CAD build for the part. Positions are in the model's coordinates, mm. A direction names the side the tool comes from. Round coordinates to 2 decimals unless told otherwise and drop trailing zeros. Loops run counter-clockwise (first coordinate to the right, second up) from the corner with the lowest first, then second, coordinate; pieces in that order, holes last.
from build123d import *

# Parameters (mm, degrees)
F0_R         = 1.5
F0_W         = 21
F0_H         = 8
F0_W_2       = 3
F0_H_2       = 5
F1_DEPTH     = 4
F2_W         = 2
F2_H         = 11
F3_DEPTH     = 1.5
F4_DEPTH     = 8
F5_T1_DEPTH  = 4
F5_T3_DEPTH  = 8
F5_T9_DEPTH  = 20.2494197933
F5_T14_DEPTH = 16.5024140205
F5_T22_DEPTH = 20.2494197933
F5_T27_DEPTH = 16.5024140205


# Not quite as in the source:
# - a fillet or chamfer that OpenCascade refuses, or shapes differently, is made with other operations: its cross-section is extruded or revolved along the edge and cut away or added


with BuildPart() as f1:
    # F0 (on Top) → F1 (new body)
    with BuildSketch(Plane.XY):
        with BuildLine():
            ThreePointArc((-3.25, 9), (0, 5.75), (3.25, 9))
            ThreePointArc((3.25, 9), (0, 12.25), (-3.25, 9))
        make_face()
        with Locations((0, 9)):
            Circle(F0_R, mode=Mode.SUBTRACT)
        with BuildLine():
            Line((3.25, -9), (3.25, 9))
            ThreePointArc((3.25, 9), (0, 5.75), (-3.25, 9))
            Line((-3.25, 9), (-3.25, 4))
            Line((-3.25, 4), (-3.25, -4))
            Line((-3.25, -4), (-3.25, -9))
            ThreePointArc((-3.25, -9), (0, -5.75), (3.25, -9))
        make_face()
        with BuildLine():
            ThreePointArc((-3.25, -9), (0, -12.25), (3.25, -9))
            ThreePointArc((3.25, -9), (0, -5.75), (-3.25, -9))
        make_face()
        with Locations((0, -9)):
            Circle(F0_R, mode=Mode.SUBTRACT)
        with Locations((-13.75, 0)):
            Rectangle(F0_W, F0_H)
        with Locations((-25.75, 0)):
            Rectangle(F0_W_2, F0_H)
        with Locations((-25.75, 6.5)):
            Rectangle(F0_W_2, F0_H_2)
        with Locations((-25.75, -6.5)):
            Rectangle(F0_W_2, F0_H_2)
    extrude(amount=F1_DEPTH)

    # F2 (on face) → F3 (cut)
    with BuildSketch(Plane.XY.offset(4)):
        Rectangle(F2_W, F2_H)
    extrude(amount=-F3_DEPTH, mode=Mode.SUBTRACT)

    # F0 (on Top) → F4 (join)
    with BuildSketch(Plane.XY):
        with Locations((-25.75, 6.5)):
            Rectangle(F0_W_2, F0_H_2)
        with Locations((-25.75, 0)):
            Rectangle(F0_W_2, F0_H)
        with Locations((-25.75, -6.5)):
            Rectangle(F0_W_2, F0_H_2)
    extrude(amount=F4_DEPTH)

    # F5: fillet of radius 5 on 3 edges, made by hand

    # F5_s2 → F5_t1 (join)
    with BuildSketch(Plane.XY):
        with BuildLine():
            ThreePointArc((-19.2490344078, 3.9996), (-22.785192534, 5.4641246619), (-24.2504, 8.9999999228))
            Line((-24.2504, 8.9999999228), (-24.7505365592, 8.9999033465))
            ThreePointArc((-24.7505365592, 8.9999033465), (-24.7501365685, 6.4999999614), (-24.7501365685, 4))
            Line((-24.7501365685, 4), (-24.25, 3.4998634315))
            ThreePointArc((-24.25, 3.4998634315), (-21.7495172039, 3.4998634315), (-19.2490344078, 3.4994634315))
            Line((-19.2490344078, 3.4994634315), (-19.2490344078, 3.9996))
        make_face()
        with BuildLine():
            ThreePointArc((-24.2504, -8.9999999228), (-22.785192534, -5.4641246619), (-19.2490344078, -3.9996))
            Line((-19.2490344078, -3.9996), (-19.2490344078, -3.4994634315))
            ThreePointArc((-19.2490344078, -3.4994634315), (-21.7495172039, -3.4998634315), (-24.25, -3.4998634315))
            Line((-24.25, -3.4998634315), (-24.7501365685, -4))
            ThreePointArc((-24.7501365685, -4), (-24.7501365685, -6.4999999614), (-24.7505365592, -8.9999033465))
            Line((-24.7505365592, -8.9999033465), (-24.2504, -8.9999999228))
        make_face()
    extrude(amount=F5_T1_DEPTH)

    # F5_s4 → F5_t3 (join)
    with BuildSketch(Plane.XZ.offset(-4)):
        with BuildLine():
            ThreePointArc((-19.350232099, 3.9996), (-22.5130680788, 5.126675133), (-24.2503919057, 7.9999199382))
            Line((-24.2503919057, 7.9999199382), (-24.7404078864, 7.8998153635))
            ThreePointArc((-24.7404078864, 7.8998153635), (-24.7501365685, 5.9999599691), (-24.7501365685, 4))
            Line((-24.7501365685, 4), (-24.25, 3.4998634315))
            ThreePointArc((-24.25, 3.4998634315), (-21.8001160495, 3.4998634315), (-19.350232099, 3.4994634315))
            Line((-19.350232099, 3.4994634315), (-19.350232099, 3.9996))
        make_face()
    extrude(amount=F5_T3_DEPTH)


with BuildPart() as f5_tool7:
    # F5_s8 → F5_t9 (new body)
    with BuildSketch(Plane.XZ.offset(-16.2494197933)):
        with BuildLine():
            ThreePointArc((-19.350232099, 3.9996), (-22.5130680788, 5.126675133), (-24.2503919057, 7.9999199382))
            Line((-24.2503919057, 7.9999199382), (-24.7404078864, 7.8998153635))
            ThreePointArc((-24.7404078864, 7.8998153635), (-24.7501365685, 5.9999599691), (-24.7501365685, 4))
            Line((-24.7501365685, 4), (-24.25, 3.4998634315))
            ThreePointArc((-24.25, 3.4998634315), (-21.8001160495, 3.4998634315), (-19.350232099, 3.4994634315))
            Line((-19.350232099, 3.4994634315), (-19.350232099, 3.9996))
        make_face()
    extrude(amount=F5_T9_DEPTH)

    split(bisect_by=Plane.XZ.offset(-4), keep=Keep.BOTTOM)

    split(bisect_by=Plane.XZ.offset(-9), keep=Keep.TOP)


with BuildPart() as f5_tool12:
    # F5_s13 → F5_t14 (new body)
    with BuildSketch(Plane.XY):
        with BuildLine():
            ThreePointArc((-19.2490344078, 3.9996), (-22.785192534, 5.4641246619), (-24.2504, 8.9999999228))
            Line((-24.2504, 8.9999999228), (-24.7505365592, 8.9999033465))
            ThreePointArc((-24.7505365592, 8.9999033465), (-24.7501365685, 6.4999999614), (-24.7501365685, 4))
            Line((-24.7501365685, 4), (-24.25, 3.4998634315))
            ThreePointArc((-24.25, 3.4998634315), (-21.7495172039, 3.4998634315), (-19.2490344078, 3.4994634315))
            Line((-19.2490344078, 3.4994634315), (-19.2490344078, 3.9996))
        make_face()
    extrude(amount=F5_T14_DEPTH)

    split(bisect_by=Plane.XY.offset(4), keep=Keep.TOP)

    split(bisect_by=Plane.XY.offset(8), keep=Keep.BOTTOM)


with BuildPart() as f5_tool7_1:
    add(f5_tool7.part)

    # F5_t17: intersect F5_tool12
    add(f5_tool12.part, mode=Mode.INTERSECT)


with BuildPart() as f1_1:
    add(f1.part)

    # F5_t5: union F5_tool7
    add(f5_tool7_1.part)


with BuildPart() as f5_tool20:
    # F5_s21 → F5_t22 (new body)
    with BuildSketch(Plane.XZ.offset(-4)):
        with BuildLine():
            ThreePointArc((-19.350232099, 3.9996), (-22.5130680788, 5.126675133), (-24.2503919057, 7.9999199382))
            Line((-24.2503919057, 7.9999199382), (-24.7404078864, 7.8998153635))
            ThreePointArc((-24.7404078864, 7.8998153635), (-24.7501365685, 5.9999599691), (-24.7501365685, 4))
            Line((-24.7501365685, 4), (-24.25, 3.4998634315))
            ThreePointArc((-24.25, 3.4998634315), (-21.8001160495, 3.4998634315), (-19.350232099, 3.4994634315))
            Line((-19.350232099, 3.4994634315), (-19.350232099, 3.9996))
        make_face()
    extrude(amount=F5_T22_DEPTH)

    split(bisect_by=Plane.XZ.offset(9), keep=Keep.BOTTOM)

    split(bisect_by=Plane.XZ.offset(4), keep=Keep.TOP)


with BuildPart() as f5_tool25:
    # F5_s26 → F5_t27 (new body)
    with BuildSketch(Plane.XY):
        with BuildLine():
            ThreePointArc((-24.2504, -8.9999999228), (-22.785192534, -5.4641246619), (-19.2490344078, -3.9996))
            Line((-19.2490344078, -3.9996), (-19.2490344078, -3.4994634315))
            ThreePointArc((-19.2490344078, -3.4994634315), (-21.7495172039, -3.4998634315), (-24.25, -3.4998634315))
            Line((-24.25, -3.4998634315), (-24.7501365685, -4))
            ThreePointArc((-24.7501365685, -4), (-24.7501365685, -6.4999999614), (-24.7505365592, -8.9999033465))
            Line((-24.7505365592, -8.9999033465), (-24.2504, -8.9999999228))
        make_face()
    extrude(amount=F5_T27_DEPTH)

    split(bisect_by=Plane.XY.offset(4), keep=Keep.TOP)

    split(bisect_by=Plane.XY.offset(8), keep=Keep.BOTTOM)


with BuildPart() as f5_tool20_1:
    add(f5_tool20.part)

    # F5_t30: intersect F5_tool25
    add(f5_tool25.part, mode=Mode.INTERSECT)


with BuildPart() as f1_2:
    add(f1_1.part)

    # F5_t18: union F5_tool20
    add(f5_tool20_1.part)


solid = f1_2.part
Item 1: Cut at C-C (z = 6). List the corners of the cut face in (x, y), plus the area to 3 significant figures.
Verdict:
outline: (-27.25, -9) - (-24.25, -9) - (-24.25, -8.94) arc R5 cw to (-23.35, -6.14) - (-23.35, 6.14) arc R5 cw to (-24.25, 8.94) - (-24.25, 9) - (-27.25, 9) - close
area: 66.7 mm2
Item 2: Cut at B-B (y = 8.5). State how many separate pieces and enclosed holes the cut face has, plus the area to 3 significant figures.
Verdict:
separate pieces: 3
enclosed holes: 0
area: 38.9 mm2
Item 3: Cut at A-A (x = 0). List the corners of the cut face in (y, z).
Verdict:
outline: (-12.25, 0) - (-10.5, 0) - (-10.5, 4) - (-12.25, 4) - close; (-7.5, 0) - (7.5, 0) - (7.5, 4) - (5.5, 4) - (5.5, 2.5) - (-5.5, 2.5) - (-5.5, 4) - (-7.5, 4) - close; (10.5, 0) - (12.25, 0) - (12.25, 4) - (10.5, 4) - close
Item 4: Mould opens along X. For faces 6 (the flat face through (0, 0, 2.5)), 7 (the flat face through (-6, 0, 4)), 8 (the cylindrical face through (-0.07, -12.25, 1.97)), 9 (the cylindrical face through (-23.048, 0.125, 5.633)) say: released by +X, released by -X, zero draft, split by the parting line, or undercut.
Verdict:
face 6: undercut
face 7: zero draft
face 8: split by the parting line
face 9: released by +X
Item 5: Wall check: L1, parallel to Y at x = 0, z = 1.3; L2, parallel to Y at x = 0, z = 2.85; L3, parallel to Z at x = 0, y = -0.5. Give the ranges that are in metal, low to high.
Verdict:
L1: y = -12.25 to -10.5, -7.5 to 7.5, 10.5 to 12.25
L2: y = -12.25 to -10.5, -7.5 to -5.5, 5.5 to 7.5, 10.5 to 12.25
L3: z = 0 to 2.5
Item 6: Cut at D-D (x = -9.5). List the corners of the cut face in (y, z).
Verdict:
outline: (-4, 0) - (4, 0) - (4, 4) - (-4, 4) - close
Item 7: 3-axis set-ups, long thin cutter, end or side, ignore diameter. For faces 1 (the flat face through (-3.25, 7, 2)), 2 (the flat face through (-26, 9, 4)), 3 (the flat face through (-3.25, -6, 2)), 4 (the flat face through (-1, 0, 3)), 5 (the flat face through (-26, -9, 4)): which of +Z, -Z, +X, -X, +Y, -Y reach the whole face in a straight line?
Verdict:
face 1: +Z, -Z, +Y
face 2: +Z, -Z, -X, +Y
face 3: +Z, -Z, -Y
face 4: +Z
face 5: +Z, -Z, -X, -Y
Item 8: Flat gauge pins, fed straight in: P1, Ø1.2, axis at x = 0.5, z = 3.5, coming from the +Y side; P2, Ø4, axis at x = -16.5, y = 4, coming from the +Z side; P3, Ø3.5, axis at x = -25.5, z = 5, coming from the -Y side; P4, Ø2, axis at x = -12, z = 1, coming from the -Y side. Where does each tip first touch, or does it go through?
Verdict:
P1: stops at y = 12.25
P2: stops at z = 4
P3: stops at y = -9
P4: stops at y = -4
